Design review of the part built by this model. Coordinates are the model's own, in mm. A direction names the side the tool comes from. Give positions to 0.01 mm unless a question says otherwise; leave off trailing zeros. Loops run counter-clockwise (first coordinate to the right, second up) from the corner with the lowest first, then second, coordinate; pieces in that order, holes last. Notation, with made-up numbers: (-7, 69) -> (29, 69) arc R26 ccw to (29, 97) -> close; hole circle Ø1 at (64.5, 14). An arc over 180 degrees is marked (long way). Answer in a Markdown table with one row per item. Add a question column.
(1) For pin 1 (3 mm diameter, centred on x = 63, z = -6, fed in from +Y), flat-tipped, find the tip position at first contact; note if it passes through.
(2) For faces 5 (the flat face through (59.323, 27, -7)), 6 (the cylindrical face through (37.7, 21.6, -1)), 7 (the flat face through (63, -19, -5.2)), 8 (the flat face through (63, -16.291, -3)), 9 (the flat face through (38, 0, -76.2)), list the 3-axis set-ups (+Z, -Z, +X, -X, +Y, -Y) from which the entire face can be reached by the end or side of a thin tool; tool diameter is ignored.
(3) Consider section A-A on x = 30.5. Write out the cut boundary in (y, z), then the cut area to 3 significant figures.
(4) Consider section D-D on x = 13.1. Write out the cut boundary in (y, z), then the cut area to 3 significant figures.
(5) For line 1 (X direction, y = -13.9, z = -3.95); line 2 (Y direction, x = 38.1, z = -0.7); line 3 (Z direction, x = 35.5, y = 31), list the stretches that pass through material, from the lowest coordinate up.
(6) Draft analysis for pull direction Y (two halves, no side actions). For faces 1 (the flat face through (50.6, 8, -75)), 2 (the cylindrical face through (21.05, 22.7, -0.99)), 3 (the flat face through (38, 20, -74.2)), 4 (the flat face through (38, -25.4, -39)), state which applies: +Y half, -Y half, draft (parallel to the pull), parting line (faces both ways), or undercut.
(7) Consider section B-B on z = -35. Write out the cut boundary in (x, y), then the cut area to 3 significant figures.
(8) Consider section C-C on y = -13.9. Write out the cut boundary in (x, z).
from build123d import *

# Parameters (mm, degrees)
SKETCH1_W           = 76.2
SKETCH1_H           = 76.2
BOSS_EXTRUDE1_DEPTH = 38.1
SHELL1_T            = -2
SKETCH2_W           = 25
SKETCH2_H           = 12
CUT_EXTRUDE1_DEPTH  = 77.2
CUT_EXTRUDE2_REACH  = 78.2
SKETCH3_R           = 4
CUT_EXTRUDE3_REACH  = 78.2
SKETCH4_R           = 6.2103
CUT_EXTRUDE4_REACH  = 78.2
SKETCH6_R           = 1.65
SKETCH1_2_W         = 76.2
SKETCH1_2_H         = 76.2
BOSS_EXTRUDE2_DEPTH = 25.4
SKETCH11_R          = 10
CUT_EXTRUDE6_DEPTH  = 71
CUT_EXTRUDE8_REACH  = 7.2
SKETCH16_W          = 51.308
SKETCH16_H          = 41.148
CUT_EXTRUDE9_DEPTH  = 1.7
BOSS_EXTRUDE3_DEPTH = 9.6774


with BuildPart() as part:
    # Sketch1 → Boss-Extrude1 (new body)
    with BuildSketch(Plane(origin=(0, 0, 0), x_dir=(1, 0, 0), z_dir=(0, 1, 0))):
        with Locations((38.1, 38.1)):
            Rectangle(SKETCH1_W, SKETCH1_H)
    extrude(amount=BOSS_EXTRUDE1_DEPTH)

    # Shell1
    shell1_openings = [part.faces().sort_by_distance(p)[0] for p in [
        (38.1, 38.1, -38.1),
    ]]
    offset(amount=SHELL1_T, openings=shell1_openings, kind=Kind.INTERSECTION)

    # Sketch2 → Cut-Extrude1 (cut, through all)
    with BuildSketch(Plane.XY):
        with Locations((38.1, 8)):
            Rectangle(SKETCH2_W, SKETCH2_H)
    extrude(amount=-CUT_EXTRUDE1_DEPTH, mode=Mode.SUBTRACT)

    # Sketch3 → Cut-Extrude2 (cut, up to next)
    with BuildSketch(Plane.XY, mode=Mode.PRIVATE) as cut_extrude2_sk1:
        with Locations((24, 20)):
            Circle(SKETCH3_R)
    cut_extrude2_tool1 = extrude(cut_extrude2_sk1.sketch, amount=-CUT_EXTRUDE2_REACH, mode=Mode.PRIVATE) & part.part
    add(cut_extrude2_tool1.solids().sort_by_distance((24, 20, 0))[0], mode=Mode.SUBTRACT)
    # Sketch3 → Cut-Extrude2 (cut, up to next)
    with BuildSketch(Plane.XY, mode=Mode.PRIVATE) as cut_extrude2_sk2:
        with Locations((8, 20)):
            Circle(SKETCH3_R)
    cut_extrude2_tool2 = extrude(cut_extrude2_sk2.sketch, amount=-CUT_EXTRUDE2_REACH, mode=Mode.PRIVATE) & part.part
    add(cut_extrude2_tool2.solids().sort_by_distance((8, 20, 0))[0], mode=Mode.SUBTRACT)
    # Sketch3 → Cut-Extrude2 (cut, up to next)
    with BuildSketch(Plane.XY, mode=Mode.PRIVATE) as cut_extrude2_sk3:
        with Locations((24, 33)):
            Circle(SKETCH3_R)
    cut_extrude2_tool3 = extrude(cut_extrude2_sk3.sketch, amount=-CUT_EXTRUDE2_REACH, mode=Mode.PRIVATE) & part.part
    add(cut_extrude2_tool3.solids().sort_by_distance((24, 33, 0))[0], mode=Mode.SUBTRACT)
    # Sketch3 → Cut-Extrude2 (cut, up to next)
    with BuildSketch(Plane.XY, mode=Mode.PRIVATE) as cut_extrude2_sk4:
        with Locations((8, 33)):
            Circle(SKETCH3_R)
    cut_extrude2_tool4 = extrude(cut_extrude2_sk4.sketch, amount=-CUT_EXTRUDE2_REACH, mode=Mode.PRIVATE) & part.part
    add(cut_extrude2_tool4.solids().sort_by_distance((8, 33, 0))[0], mode=Mode.SUBTRACT)

    # Sketch4 → Cut-Extrude3 (cut, up to next)
    with BuildSketch(Plane.XY, mode=Mode.PRIVATE) as cut_extrude3_sk1:
        with Locations((65.8, 24.5)):
            Circle(SKETCH4_R)
    cut_extrude3_tool1 = extrude(cut_extrude3_sk1.sketch, amount=-CUT_EXTRUDE3_REACH, mode=Mode.PRIVATE) & part.part
    add(cut_extrude3_tool1.solids().sort_by_distance((65.8, 24.5, 0))[0], mode=Mode.SUBTRACT)

    # Sketch6 → Cut-Extrude4 (cut, up to next)
    with BuildSketch(Plane.XY, mode=Mode.PRIVATE) as cut_extrude4_sk1:
        with Locations((38.1, 23.2)):
            Circle(SKETCH6_R)
    cut_extrude4_tool1 = extrude(cut_extrude4_sk1.sketch, amount=-CUT_EXTRUDE4_REACH, mode=Mode.PRIVATE) & part.part
    add(cut_extrude4_tool1.solids().sort_by_distance((38.1, 23.2, 0))[0], mode=Mode.SUBTRACT)
    # Sketch6 → Cut-Extrude4 (cut, up to next)
    with BuildSketch(Plane.XY, mode=Mode.PRIVATE) as cut_extrude4_sk2:
        with Locations((38.1, 33.2)):
            Circle(SKETCH6_R)
    cut_extrude4_tool2 = extrude(cut_extrude4_sk2.sketch, amount=-CUT_EXTRUDE4_REACH, mode=Mode.PRIVATE) & part.part
    add(cut_extrude4_tool2.solids().sort_by_distance((38.1, 33.2, 0))[0], mode=Mode.SUBTRACT)

    # Sketch1_2 → Boss-Extrude2 (add)
    with BuildSketch(Plane(origin=(0, 0, 0), x_dir=(1, 0, 0), z_dir=(0, 1, 0))):
        with Locations((38.1, 38.1)):
            Rectangle(SKETCH1_2_W, SKETCH1_2_H)
    extrude(amount=-BOSS_EXTRUDE2_DEPTH)

    # Sketch11 → Cut-Extrude6 (cut)
    with BuildSketch(Plane(origin=(0, 0, -76.2), x_dir=(-1, 0, 0), z_dir=(0, 0, -1))):
        with Locations((-63.1, -13.9)):
            Circle(SKETCH11_R)
        with Locations((-13.1, -13.9)):
            Circle(SKETCH11_R)
    extrude(amount=-CUT_EXTRUDE6_DEPTH, mode=Mode.SUBTRACT)

    # Sketch15 → Cut-Extrude8 (cut, up to next)
    with BuildSketch(Plane(origin=(0, 0, -5.2), x_dir=(-1, 0, 0), z_dir=(0, 0, -1)), mode=Mode.PRIVATE) as cut_extrude8_sk1:
        with BuildLine():
            Line((-72.809962586, -16.290946797), (-53.390037414, -16.290946797))
            ThreePointArc((-53.390037414, -16.290946797), (-63.1, -3.9), (-72.809962586, -16.290946797))
        make_face()
    cut_extrude8_tool1 = extrude(cut_extrude8_sk1.sketch, amount=-CUT_EXTRUDE8_REACH, mode=Mode.PRIVATE) & part.part
    add(cut_extrude8_tool1.solids().sort_by_distance((63.1, -10.914633, -5.2))[0], mode=Mode.SUBTRACT)
    # Sketch15 → Cut-Extrude8 (cut, up to next)
    with BuildSketch(Plane(origin=(0, 0, -5.2), x_dir=(-1, 0, 0), z_dir=(0, 0, -1)), mode=Mode.PRIVATE) as cut_extrude8_sk2:
        with BuildLine():
            Line((-22.809962586, -16.290946797), (-3.390037414, -16.290946797))
            ThreePointArc((-3.390037414, -16.290946797), (-13.1, -3.9), (-22.809962586, -16.290946797))
        make_face()
    cut_extrude8_tool2 = extrude(cut_extrude8_sk2.sketch, amount=-CUT_EXTRUDE8_REACH, mode=Mode.PRIVATE) & part.part
    add(cut_extrude8_tool2.solids().sort_by_distance((13.1, -10.914633, -5.2))[0], mode=Mode.SUBTRACT)

    # Sketch16 → Cut-Extrude9 (cut)
    with BuildSketch(Plane(origin=(0, 2, 0), x_dir=(1, 0, 0), z_dir=(0, 1, 0))):
        with Locations((35.046, 22.574)):
            Rectangle(SKETCH16_W, SKETCH16_H)
    extrude(amount=-CUT_EXTRUDE9_DEPTH, mode=Mode.SUBTRACT)

    # Sketch19 → Boss-Extrude3 (add)
    with BuildSketch(Plane(origin=(0, 0, -2), x_dir=(-1, 0, 0), z_dir=(0, 0, -1))):
        Polygon((-59.323, 34.9267), (-59.323, 18.1867), (-72.277, 18.1867), (-72.277, 34.9267), (-74.2, 34.9267), (-74.2, 15.742753149), (-57.2, 15.742753149), (-57.2, 34.9267), align=None)
    extrude(amount=BOSS_EXTRUDE3_DEPTH)


solid = part.part
Values follow:
| question | item | result |
|---|---|---|
| 1 | pin 1 | y = 18.19 |
| 2 | face 5 | +Y |
| 2 | face 6 | +Z |
| 2 | face 7 | -Z |
| 2 | face 8 | +Z, -Z |
| 2 | face 9 | -Z, +X, -X, +Y, -Y |
| 3 | outline | (-25.4, -76.2) -> (2, -76.2) -> (2, -43.15) -> (0.3, -43.15) -> (0.3, -2) -> (2, -2) -> (2, 0) -> (-25.4, 0) -> close; (14, -76.2) -> (38.1, -76.2) -> (38.1, -74.2) -> (14, -74.2) -> close; (14, -2) -> (38.1, -2) -> (38.1, 0) -> (14, 0) -> close |
| 3 | area | 2,110 mm2 |
| 4 | outline | (-25.4, -76.2) -> (-23.9, -76.2) -> (-23.9, -5.2) -> (-16.29, -5.2) -> (-16.29, 0) -> (-25.4, 0) -> close; (-3.9, -76.2) -> (38.1, -76.2) -> (38.1, -74.2) -> (2, -74.2) -> (2, -43.15) -> (0.3, -43.15) -> (0.3, -2) -> (38.1, -2) -> (38.1, 0) -> (-3.9, 0) -> close |
| 4 | area | 678 mm2 |
| 5 | line 1 | 0 to 3.1, 23.1 to 53.1, 73.1 to 76.2 |
| 5 | line 2 | -25.4 to 2, 14 to 21.55, 24.85 to 31.55, 34.85 to 38.1 |
| 5 | line 3 | -76.2 to -74.2, -2 to 0 |
| 6 | face 1 | undercut |
| 6 | face 2 | undercut |
| 6 | face 3 | draft |
| 6 | face 4 | -Y half |
| 7 | outline | (0, -25.4) -> (76.2, -25.4) -> (76.2, 38.1) -> (74.2, 38.1) -> (74.2, 2) -> (60.7, 2) -> (60.7, 0.3) -> (9.39, 0.3) -> (9.39, 2) -> (2, 2) -> (2, 38.1) -> (0, 38.1) -> close; hole circle Ø20 at (13.1, -13.9); hole circle Ø20 at (63.1, -13.9) |
| 7 | area | 1,520 mm2 |
| 8 | outline | (0, -76.2) -> (3.1, -76.2) -> (3.1, 0) -> (0, 0) -> close; (23.1, -76.2) -> (53.1, -76.2) -> (53.1, 0) -> (23.1, 0) -> close; (73.1, -76.2) -> (76.2, -76.2) -> (76.2, 0) -> (73.1, 0) -> close |
